```python
from build123d import *

# Parameters (mm, degrees)
F0_R     = 15.259541
F1_DEPTH = 25.4
F2_SIZE  = 5.08


with BuildPart() as f1:
    # F0 (on Top) → F1 (new body)
    with BuildSketch(Plane.XY):
        Polygon((-58.197681, 34.701545), (-128.283679, 0), (-119.025573, -54.748576), (4.151391, -11.995041), align=None)
        with Locations((-77.978395, -3.722796)):
            Circle(F0_R, mode=Mode.SUBTRACT)
    extrude(amount=F1_DEPTH)

    # F2
    f2_edges = [f1.edges().sort_by_distance(p)[0] for p in [
        (-93.24068, 17.350772, 25.4),
        (-123.654626, -27.374288, 25.4),
        (-57.437091, -33.371808, 25.4),
        (-27.023145, 11.353252, 25.4),
    ]]
    chamfer(f2_edges, length=F2_SIZE)


solid = f1.part
```
Verification items for the finished model (mm, model axes). Round coordinates to 2 decimals unless told otherwise and drop trailing zeros. Order: outer loops, then holes, each group sorted by start corner. A loop starts at its lowest first (then second) coordinate and runs counter-clockwise, first axis right, second up. Notation, with made-up numbers: (33.25, 29.25) - (85.25, 29.25) arc R27 ccw to (85.25, 67.25) - close; hole circle Ø5 at (60, 23). An arc over 180 degrees is marked (long way). Use CSV: the item, a comma, the result in double quotes. Start each with the question number.
1) Section check D-D, the plane x = -109. Record the cut outline in (y, z), plus the area to 3 significant figures.
2) Thickness scan on L1, parallel to Y at x = -86.5, z = 2.5; L2, parallel to Y at x = -78.5, z = 15.75; L3, parallel to X at y = 4.5, z = 22. Record the ranges inside material, lowest first.
3) Go/stop test with flat-tipped pins: P1, Ø5, axis at y = -0.5, z = 12, coming from the +X side; P2, Ø1, axis at y = -27.5, z = 7, coming from the -X side; P3, Ø2, axis at x = -72.5, z = 8, coming from the -Y side. Record where each tip stops, or that it passes through.
4) Section check B-B, the plane y = -8. Record the cut outline in (x, z).
5) Mould release check, pull along X, two halves, no side actions. Record for faces 1 (the flat face through (-26.59, 11.03, 10.02)), 2 (the cylindrical face through (-63.424, 0.861, 12.522)), 3 (the flat face through (-123.72, -26.99, 10.02)): +X half, -X half, draft (parallel to the pull), parting line (faces both ways), or undercut.
6) Section check A-A, the plane x = -68.5. Record the cut outline in (y, z), plus the area to 3 significant figures.
7) Section check C-C, the plane z = 7. Record the cut outline in (x, y), plus the area to 3 significant figures.
Answers:
1,outline,"(-51.27, 0) - (9.55, 0) - (9.55, 20.32) - (3.88, 25.4) - (-45.89, 25.4) - (-51.27, 20.32) - close"
1,area,"1,520 mm²"
2,L1,"y = -43.46 to -16.38, 8.94 to 20.69"
2,L2,"y = -40.68 to -18.97, 11.53 to 24.65"
2,L3,"x = -115.41 to -90.83, -65.12 to -20.68"
3,P1,"stops at x = -7.86"
3,P2,"stops at x = -123.72"
3,P3,"stops at y = -38.95"
4,outline,"(-126.93, 0) - (-92.63, 0) - (-92.63, 25.4) - (-121.78, 25.4) - (-126.93, 20.32) - close; (-63.33, 0) - (-1.18, 0) - (-1.18, 20.32) - (-9.66, 25.4) - (-63.33, 25.4) - close"
5,face 1,"+X half"
5,face 2,"undercut"
5,face 3,"-X half"
6,outline,"(-37.21, 0) - (-15.68, 0) - (-15.68, 25.4) - (-31.83, 25.4) - (-37.21, 20.32) - close; (8.24, 0) - (29.6, 0) - (29.6, 20.32) - (23.93, 25.4) - (8.24, 25.4) - close"
6,area,"1,060 mm²"
7,outline,"(-128.28, 0) - (-119.03, -54.75) - (4.15, -12) - (-58.2, 34.7) - close; hole circle Ø30.52 at (-77.98, -3.72)"
7,area,"5,560 mm²"
